from build123d import *

# Parameters (mm, degrees)
BOSS_EXTRUDE1_DEPTH                            = 40
CUT_EXTRUDE1_DEPTH                             = 40
CSK_FOR_M5_FLAT_HEAD_MACHINE_SCREW1_AT_2_COUNT = 2
CSK_FOR_M5_FLAT_HEAD_MACHINE_SCREW1_AT_2_PITCH = 25
SKETCH7_R                                      = 2
CUT_EXTRUDE2_DEPTH                             = 40
SKETCH8_W                                      = 1
SKETCH8_H                                      = 10.2
CUT_EXTRUDE3_DEPTH                             = 10
SKETCH9_W                                      = 11.70124712
SKETCH9_H                                      = 10.2
CUT_EXTRUDE4_DEPTH                             = 10
CUT_EXTRUDE4_DEPTH_BACK                        = 10
SKETCH10_W                                     = 1
SKETCH10_H                                     = 10
CUT_EXTRUDE5_DEPTH                             = 10
SKETCH11_W                                     = 12.165826364
SKETCH11_H                                     = 10.874220792
CUT_EXTRUDE6_DEPTH                             = 10
CUT_EXTRUDE6_DEPTH_BACK                        = 10


with BuildPart() as part:
    # Sketch2 → Boss-Extrude1 (new body)
    with BuildSketch(Plane(origin=(0, 0, 0), x_dir=(1, 0, 0), z_dir=(0, 1, 0))):
        with BuildLine():
            Line((-2.5, 0), (2.5, 0))
            Line((2.5, 0), (5, 2.5))
            Line((5, 2.5), (5, 4))
            Line((5, 4), (20, 4))
            Line((20, 4), (20, 9))
            Line((20, 9), (6, 9))
            Line((6, 9), (6, 8.5))
            Line((6, 8.5), (0, 8.5))
            ThreePointArc((0, 8.5), (-3.535533906, 7.035533906), (-5, 3.5))
            Line((-5, 3.5), (-5, 2.5))
            Line((-5, 2.5), (-2.5, 0))
        make_face()
    extrude(amount=BOSS_EXTRUDE1_DEPTH)

    # Sketch3 → Cut-Extrude1 (cut)
    with BuildSketch(Plane(origin=(0, 40, 0), x_dir=(1, 0, 0), z_dir=(0, 1, 0))):
        Polygon((20, 6.5), (18.56, 4), (20, 4), align=None)
    extrude(amount=-CUT_EXTRUDE1_DEPTH, mode=Mode.SUBTRACT)

    # Sketch6 → CSK for M5 Flat Head Machine Screw1 (revolve, cut)
    with BuildSketch(Plane(origin=(12.5, 32.5, -4), x_dir=(0, -1, 0), z_dir=(1, 0, 0))):
        Polygon((0, 0), (0, 5), (2.65, 5), (2.65, 2.55), (5.2, 0), align=None)
    csk_for_m5_flat_head_machine_screw1 = revolve(axis=Axis((12.5, 32.5, 2.35), (0, 0, -1)), mode=Mode.SUBTRACT)

    # CSK for M5 Flat Head Machine Screw1 at 2: CSK for M5 Flat Head Machine Screw1 ×2
    with Locations(*[(0, -i * CSK_FOR_M5_FLAT_HEAD_MACHINE_SCREW1_AT_2_PITCH, 0) for i in range(1, CSK_FOR_M5_FLAT_HEAD_MACHINE_SCREW1_AT_2_COUNT)]):
        add(csk_for_m5_flat_head_machine_screw1, mode=Mode.SUBTRACT)

    # Sketch7 → Cut-Extrude2 (cut)
    with BuildSketch(Plane(origin=(0, 40, 0), x_dir=(1, 0, 0), z_dir=(0, 1, 0))):
        with Locations((0, 3.5)):
            Circle(SKETCH7_R)
    extrude(amount=-CUT_EXTRUDE2_DEPTH, mode=Mode.SUBTRACT)

    # Sketch8 → Cut-Extrude3 (cut)
    with BuildSketch(Plane.XY.offset(-4)):
        with Locations((5.5, 25)):
            Rectangle(SKETCH8_W, SKETCH8_H)
    extrude(amount=-CUT_EXTRUDE3_DEPTH, mode=Mode.SUBTRACT)

    # Sketch9 → Cut-Extrude4 (cut, two sides)
    with BuildSketch(Plane.XY.offset(-4)) as cut_extrude4_sk:
        with Locations((0.14937644, 25)):
            Rectangle(SKETCH9_W, SKETCH9_H)
    extrude(amount=CUT_EXTRUDE4_DEPTH, mode=Mode.SUBTRACT)
    extrude(cut_extrude4_sk.sketch, amount=-CUT_EXTRUDE4_DEPTH_BACK, mode=Mode.SUBTRACT)

    # Sketch10 → Cut-Extrude5 (cut)
    with BuildSketch(Plane.XY.offset(-4)):
        with Locations((5.5, 5)):
            Rectangle(SKETCH10_W, SKETCH10_H)
    extrude(amount=-CUT_EXTRUDE5_DEPTH, mode=Mode.SUBTRACT)

    # Sketch11 → Cut-Extrude6 (cut, two sides)
    with BuildSketch(Plane.XY.offset(-4)) as cut_extrude6_sk:
        with Locations((-0.082913182, 4.562889604)):
            Rectangle(SKETCH11_W, SKETCH11_H)
    extrude(amount=CUT_EXTRUDE6_DEPTH, mode=Mode.SUBTRACT)
    extrude(cut_extrude6_sk.sketch, amount=-CUT_EXTRUDE6_DEPTH_BACK, mode=Mode.SUBTRACT)


solid = part.part
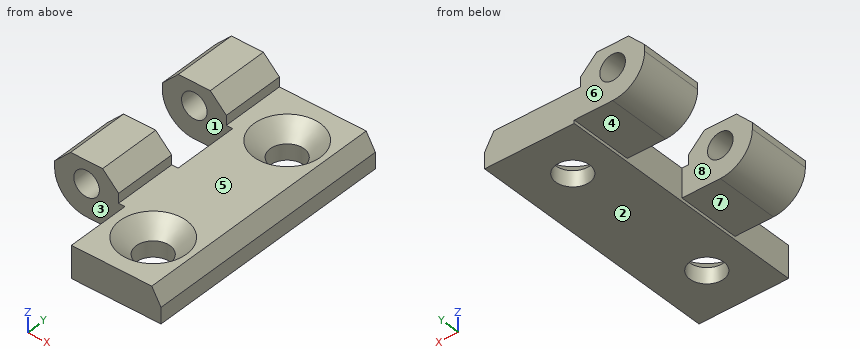
Design review of the part built by this model. Coordinates are the model's own, in mm. Face numbers are marked on the shaded views. A direction names the side the tool comes from. Coordinates: 2 decimals unless noted, no trailing zeros. Write each loop counter-clockwise with the first axis right and the second up, starting at its lowest first coordinate (ties: lowest second). Pieces come first, ordered by that corner, then holes. Notation, with made-up numbers: (82, 28) - (112, 28) arc R31 ccw to (112, 53) - close; hole circle Ø3 at (78, -29). An arc over 180 degrees is marked (long way). One line per item, written item: value.
1) Add section A-A (y = 32.5). State the section outline as (x, z) points.
Answer sheet:
outline: (-5, -3.5) arc R5 ccw to (0, -8.5) - (6, -8.5) - (6, -9) - (9.85, -9) - (9.85, -6.55) - (7.3, -4) - (5, -4) - (5, -2.5) - (2.5, 0) - (-2.5, 0) - (-5, -2.5) - close; (15.15, -9) - (20, -9) - (20, -6.5) - (18.56, -4) - (17.7, -4) - (15.15, -6.55) - close; hole circle Ø4 at (0, -3.5)
2) Add section C-C (z = -5). State the section outline as (x, y) points, plus the area to 3 significant figures.
Answer sheet:
outline: (-4.77, 10) - (-1.32, 10) - (-1.32, 19.9) - (-4.77, 19.9) - close; (-4.77, 30.1) - (-1.32, 30.1) - (-1.32, 40) - (-4.77, 40) - close; (1.32, 10) - (6, 10) - (6, 0) - (19.14, 0) - (19.14, 40) - (1.32, 40) - (1.32, 30.1) - (6, 30.1) - (6, 19.9) - (1.32, 19.9) - close; hole circle Ø8.4 at (12.5, 7.5); hole circle Ø8.4 at (12.5, 32.5)
area: 575 mm2
3) For the marked faces 1, 2, 3, 4 and 5, list the 3-axis set-ups (+Z, -Z, +X, -X, +Y, -Y) from which the entire face can be reached by the end or side of a thin tool; tool diameter is ignored.
Answer sheet:
face 1: +Z, -Z, -X
face 2: -Z, +X, -X, +Y, -Y
face 3: +Z, -Z, -X, -Y
face 4: -Z, -X, +Y, -Y
face 5: +Z, +X, +Y, -Y
4) Add section D-D (y = 17). State the section outline as (x, z) points.
Answer sheet:
outline: (-5, -3.5) arc R5 ccw to (0, -8.5) - (6, -8.5) - (6, -9) - (20, -9) - (20, -6.5) - (18.56, -4) - (5, -4) - (5, -2.5) - (2.5, 0) - (-2.5, 0) - (-5, -2.5) - close; hole circle Ø4 at (0, -3.5)
5) Mouldability with a two-part tool opening along Y and no side actions: class the marked faces 6, 7 and 8 as +Y half, -Y half, draft (parallel to the pull), parting line (faces both ways), or undercut.
Answer sheet:
face 6: +Y half
face 7: draft
face 8: undercut
6) Add section B-B (x = 12.5). State the section outline as (y, z) points.
Answer sheet:
outline: (0, -9) - (4.85, -9) - (4.85, -6.55) - (2.3, -4) - (0, -4) - close; (10.15, -9) - (29.85, -9) - (29.85, -6.55) - (27.3, -4) - (12.7, -4) - (10.15, -6.55) - close; (35.15, -9) - (40, -9) - (40, -4) - (37.7, -4) - (35.15, -6.55) - close
7) To check wall thickness, follow probe 1 along Y at (x, z) = (12.5, -7.95); probe 2 along X at (y, z) = (17, -3.5); probe 3 along Y at (x, z) = (3.75, -4.5). State the ranges of each line that lie inside material, in increasing order.
Answer sheet:
probe 1: y = 0 to 4.85, 10.15 to 29.85, 35.15 to 40
probe 2: x = -5 to -2, 2 to 5
probe 3: y = 10 to 19.9, 30.1 to 40
8) Insertion check: pin 1 (2 mm diameter, centred on y = 8.5, z = -7.5, fed in from -X); pin 2 (6 mm diameter, centred on x = 12.5, y = 7.5, fed in from +Z); pin 3 (1.6 mm diameter, centred on y = 35.5, z = -3.5, fed in from +X); pin 4 (3 mm diameter, centred on x = 0, z = -3.5, fed in from -Y). Each pin has a flat end and moves straight along its axis. Give the tip position at first contact, or say it passes through.
Answer sheet:
pin 1: stops at x = 6
pin 2: stops at z = -6.2
pin 3: stops at x = 18.73
pin 4: passes through
